Autodesk Inventor part; units mm, degrees
ref_plane "Work Plane1" through (14.1026, -8.3728, 0) normal (0, 0, 1) x (0.9999, -0.0156, 0)
ref_plane "Work Plane2" through (-268.3983, -269.3131, 111.1682) normal (0, 0, -1) x (0, 1, 0)
ref_plane "YZ Plane" through (0, 0, 0) normal (1, 0, 0) x (0, 1, 0)
ref_plane "Work Plane1" through (14.1026, -8.3728, 0) normal (0, 0, 1) x (0.9999, -0.0156, 0)
sketch "Sketch1" plane through (14.1026, -8.3728, 0) normal (0, 0, 1) x (0.9999, -0.0156, 0)
  circle A0 centre (-133.5116, -35.2578) radius 2.794
  circle A1 centre (-7.1362, -123.2288) radius 2.286 construction
  circle A2 centre (-67.2141, -131.9038) radius 3.9624 construction
  circle A3 centre (-44.9289, -42.7619) radius 2.286
  arc A4 (-133.5116, -35.2578) -> (-7.1362, -123.2288) centre (-44.9289, -42.7619) ccw construction
  arc A5 (-113.6145, -38.2305) -> (-113.6145, -38.2305) centre (-133.5116, -35.2578) ccw
  arc A6 (-5.1205, -129.2504) -> (-5.1205, -129.2504) centre (-7.1362, -123.2288) ccw
  arc A7 (-133.5116, -35.2578) -> (-7.1362, -123.2288) centre (-44.9289, -42.7619) ccw construction
  arc A8 (-138.5735, -34.829) -> (-4.9766, -127.8269) centre (-44.9289, -42.7619) ccw
  arc A9 (-128.4497, -35.6866) -> (-9.2958, -118.6307) centre (-44.9289, -42.7619) ccw
  arc A10 (-128.4497, -35.6866) -> (-138.5735, -34.829) centre (-133.5116, -35.2578) ccw
  arc A11 (-4.9766, -127.8269) -> (-9.2958, -118.6307) centre (-7.1362, -123.2288) ccw
  point P0 (-14.2313, 8.1521)
  dimension "d0" = 12.7
  dimension "d3" = 10.16
ref_plane "Work Plane2" through (-268.3983, -269.3131, 111.1682) normal (0, 0, -1) x (0, 1, 0)
extrude "Extrusion1" add sketch "Sketch1" along normal up to surface (111.1682 mm away) contours A8 A10 A9 A5 | A5 A9 A6 A8 | A6 A9 A11 A8 picked at (-134.0145, -50.6087) picked at (-9.8396, -124.4417)
properties part number "Mesh"
For this review, take the finished solid that the model builds, in its own axes (mm). Round coordinates to 2 decimals unless told otherwise and drop trailing zeros. Write each loop counter-clockwise with the first axis right and the second up, starting at its lowest first coordinate (ties: lowest second). Pieces come first, ordered by that corner, then holes. Notation, with made-up numbers: (-15, 58) -> (42, 58) arc R14 ccw to (42, 74) -> close; hole circle Ø9 at (13.5, 56.5). An arc over 180 degrees is marked (long way). Put each result on its own line as item: value.
Q1. Consider section A-A on x = -6. State the section outline as (y, z) points.
Determined:
outline: (-140.89, 0) -> (-130.28, 0) -> (-130.28, 111.17) -> (-140.89, 111.17) -> close
Q2. Clearance check with flat-ended pins moving along their axes: pin 1 Ø6 at (x, z) = (-48, 78.5) entering from -Y; pin 2 Ø10 at (x, z) = (-72.5, 20) entering from +Y; pin 3 Ø1 at (x, z) = (-52.5, 28.5) entering from +Y; pin 4 Ø3.5 at (x, y) = (-119.94, -41.54) entering from -Z. State where each tip first meets the part, or that it passes through.
Determined:
pin 1: stops at y = -143.43
pin 2: stops at y = -120.49
pin 3: stops at y = -131.44
pin 4: passes through
Q3. Consider section B-B on y = -59.5. State the section outline as (x, z) points.
Determined:
outline: (-125.03, 0) -> (-114.82, 0) -> (-114.82, 111.17) -> (-125.03, 111.17) -> close
Q4. To check wall thickness, follow L1, parallel to X at y = -48.5, z = 69; L2, parallel to Y at x = -30, z = 65; L3, parallel to X at y = -50, z = 98. State the ranges of each line that lie inside material, in increasing order. Write a range as [from, to].
Determined:
L1: x = [-125.45, -115.29]
L2: y = [-144.4, -134.24]
L3: x = [-125.47, -115.31]
